Part print with two shaded views. Sizes in mm from the minimum x, y, z corner. Round coordinates to 2 decimals unless told otherwise and drop trailing zeros. Order: outer loops, then holes, each group sorted by start corner. A loop starts at its lowest first (then second) coordinate and runs counter-clockwise, first axis right, second up. Notation, with made-up numbers: M 46.5,88 L 89.5,88 A19 cw 89.5,113 Z; hole C 74,5.25 d1. An arc over 180 degrees is marked long. One line per question, with ' | ' between items.
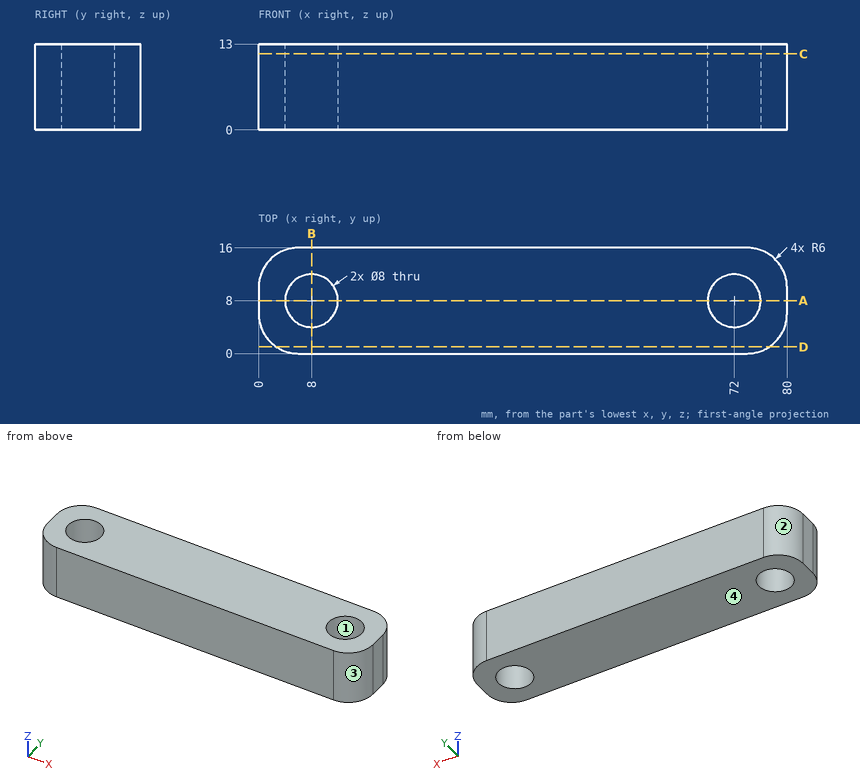
1) Probe line 1 (X direction, y = 8, z = 6.5); line 2 (Y direction, x = 72, z = 3.75); line 3 (X direction, y = 7.25, z = 6.5). List the from-to ranges inside material, lowest first. Write a range as [from, to].
The answers:
line 1: x = [0, 4], [12, 68], [76, 80] | line 2: y = [0, 4], [12, 16] | line 3: x = [0, 4.07], [11.93, 68.07], [75.93, 80]
2) Saw through at A-A (y = 8). List the corners of the cut face in (x, z).
The answers:
outline: M 0,0 L 4,0 L 4,13 L 0,13 Z; M 12,0 L 68,0 L 68,13 L 12,13 Z; M 76,0 L 80,0 L 80,13 L 76,13 Z
3) Two-plate mould, pull along X, no slides. Class the marked faces 1, 2, 3 and 4: released by +X, released by -X, zero draft, split by the parting line, or undercut.
The answers:
face 1: undercut | face 2: released by -X | face 3: released by +X | face 4: zero draft
4) Saw through at C-C (z = 11.5). List the corners of the cut face in (x, y), plus the area to 3 significant figures.
The answers:
outline: M 0,6 A6 ccw 6,0 L 74,0 A6 ccw 80,6 L 80,10 A6 ccw 74,16 L 6,16 A6 ccw 0,10 Z; hole C 8,8 d8; hole C 72,8 d8 | area: 1,150 mm²
5) Saw through at B-B (x = 8). List the corners of the cut face in (y, z).
The answers:
outline: M 0,0 L 4,0 L 4,13 L 0,13 Z; M 12,0 L 16,0 L 16,13 L 12,13 Z
6) Saw through at D-D (y = 1). List the corners of the cut face in (x, z).
The answers:
outline: M 2.68,0 L 77.32,0 L 77.32,13 L 2.68,13 Z
